Geometry check sheet. Reference: the model listing, model coordinates, mm. Face numbers are marked on the shaded views. A direction names the side the tool comes from. Coordinates: 2 decimals unless noted, no trailing zeros. Order: outer loops, then holes, each group sorted by start corner. A loop starts at its lowest first (then second) coordinate and runs counter-clockwise, first axis right, second up.
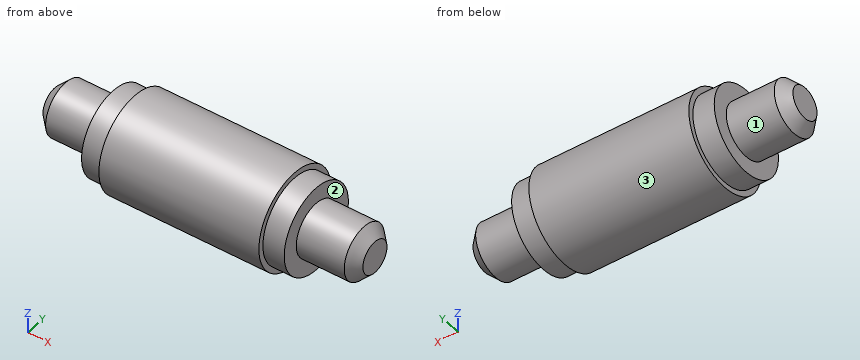
Autodesk Inventor part; units mm, degrees
ref_plane "YZ Plane" through (0, 0, 0) normal (1, 0, 0) x (0, 1, 0)
ref_plane "XZ Plane" through (0, 0, 0) normal (0, 1, 0) x (-1, 0, 0)
ref_plane "XY Plane" through (0, 0, 0) normal (0, 0, 1) x (1, 0, 0)
sketch "Náčrt1" plane through (0, 0, 0) normal (0, 0, 1) x (1, 0, 0)
  line L0 (0, 0) -> (0, 5)
  line L1 (0, 5) -> (11, 5)
  line L2 (11, 5) -> (11, 8)
  line L3 (11, 8) -> (15, 8)
  line L4 (15, 8) -> (15, 9)
  line L5 (15, 9) -> (45, 9)
  line L6 (45, 9) -> (45, 8)
  line L7 (45, 8) -> (49, 8)
  line L8 (49, 8) -> (49, 5)
  line L9 (49, 5) -> (60, 5)
  line L10 (60, 5) -> (60, 0)
  line L11 (60, 0) -> (0, 0)
  dimension "d0" = 11
  dimension "d1" = 15
  dimension "d2" = 10
  dimension "d3" = 16
  dimension "d4" = 18
  dimension "d5" = 45
revolve "Rotace1" add sketch "Náčrt1" angle 360 about axis through (60, 0, 0) along (-1, 0, 0)
chamfer "Zkosení1" distance 2 angle 45 2 edges at (0, -5, 0) (60, -5, 0)
thread "Závit1"
thread "Závit2"
properties part number "čep háku"
Item 1: Sectioned sample at D-D (z = -5.75). Record the cut outline in (x, y), and give its area (3 significant figures).
Item 2: Sectioned sample at A-A (y = 0). Record the cut outline in (x, z).
Item 3: Sectioned sample at C-C (x = 13.5). Record the cut outline in (y, z).
Item 4: Depth check by flat-ended pin: P1, Ø3, axis at x = 14.5, z = 4, coming from the -Y side; P2, Ø3, axis at x = 23, y = 6, coming from the +Z side; P3, Ø5, axis at x = 42, y = -7, coming from the -Z side. Enter the tip coordinate at first touch or a pass-through.
Item 5: Thickness scan on line 1 along X through (y, z) = (-5.75, -0.75); line 2 along Z through (x, y) = (47.5, 0); line 3 along X through (y, z) = (5.75, -6.25). Record the ranges inside material, lowest first.
Item 6: Tool access check on the marked faces 1, 2 and 3. Record the directions out of +Z, -Z, +X, -X, +Y, -Y that give a thin tool (end or side, any length) a straight path to the whole face; none if there is none.
Geometry check:
1. outline: (11, -5.56) - (15, -5.56) - (15, -6.92) - (45, -6.92) - (45, -5.56) - (49, -5.56) - (49, 5.56) - (45, 5.56) - (45, 6.92) - (15, 6.92) - (15, 5.56) - (11, 5.56) - close
1. area: 504 mm2
2. outline: (0, -3) - (2, -5) - (11, -5) - (11, -8) - (15, -8) - (15, -9) - (45, -9) - (45, -8) - (49, -8) - (49, -5) - (58, -5) - (60, -3) - (60, 3) - (58, 5) - (49, 5) - (49, 8) - (45, 8) - (45, 9) - (15, 9) - (15, 8) - (11, 8) - (11, 5) - (2, 5) - (0, 3) - close
3. outline: circle Ø16 at (0, 0)
4. P1: stops at y = -8.62
4. P2: stops at z = 7.79
4. P3: stops at z = -7.79
5. line 1: x = 11 to 49
5. line 2: z = -8 to 8
5. line 3: x = 15 to 45
6. face 1: -X
6. face 2: +X
6. face 3: +X, -X
